from build123d import *

# Parameters (mm, degrees)
F0_R     = 43.4000447198
F1_DEPTH = 110.744
F2_T     = -5.08
F3_R     = 63.6187489092
F4_DEPTH = 5.842
F5_R     = 5.07999
F6_W     = 2.7671808675
F6_H     = 25.928324776
F7_DEPTH = 50.8


# Not quite as in the source:
# - a fillet or chamfer is up to 0.001 mm smaller than in the source, because OpenCascade refuses the exact size


with BuildPart() as f1:
    # F0 (on Top) → F1 (new body)
    with BuildSketch(Plane.XY):
        Circle(F0_R)
    extrude(amount=F1_DEPTH)

    # F2
    f2_openings = [f1.faces().sort_by_distance(p)[0] for p in [
        (0, 0, 110.744),
    ]]
    offset(amount=F2_T, openings=f2_openings)

    # F3 (on Top) → F4 (join)
    with BuildSketch(Plane.XY):
        Circle(F3_R)
    extrude(amount=F4_DEPTH)

    # F5 (radius 5.08 in the source; OpenCascade refuses exactly that, so slightly less here)
    f5_edges = [f1.edges().sort_by_distance(p)[0] for p in [
        (-43.400045, 0, 110.744),
    ]]
    fillet(f5_edges, radius=F5_R)

    # F6 (on Top) → F7 (join)
    with BuildSketch(Plane.XY):
        with BuildLine():
            ThreePointArc((22.0028883346, -9.7789997235), (23.5536000152, -4.9983854371), (24.0781214104, 0))
            ThreePointArc((24.0781214104, 0), (23.5424460635, 5.0506597592), (21.9592547789, 9.8765915281))
            Line((21.9592547789, 9.8765915281), (21.9592547789, -9.7789997235))
            Line((21.9592547789, -9.7789997235), (22.0028883346, -9.7789997235))
        make_face()
        with BuildLine():
            ThreePointArc((21.9592547789, 9.8765915281), (23.5424460635, 5.0506597592), (24.0781214104, 0))
            ThreePointArc((24.0781214104, 0), (23.5536000152, -4.9983854371), (22.0028883346, -9.7789997235))
            Line((22.0028883346, -9.7789997235), (24.7264356464, -9.7789997235))
            Line((24.7264356464, -9.7789997235), (24.7264356464, 16.1493250525))
            Line((24.7264356464, 16.1493250525), (21.9592547789, 16.1493250525))
            Line((21.9592547789, 16.1493250525), (21.9592547789, 9.8765915281))
        make_face()
        with BuildLine():
            Line((21.9592547789, -9.7789997235), (21.9592547789, 9.8765915281))
            ThreePointArc((21.9592547789, 9.8765915281), (2.7373131328, 23.9220201377), (-19.1605677938, 14.5817890698))
            Line((-19.1605677938, 14.5817890698), (-19.1165860754, 14.5817890698))
            Line((-19.1165860754, 14.5817890698), (-19.1165860754, 4.2168572654))
            Line((-19.1165860754, 4.2168572654), (-6.283051686, 4.2168572654))
            Line((-6.283051686, 4.2168572654), (-6.283051686, 14.5817890698))
            Line((-6.283051686, 14.5817890698), (-3.4518897579, 14.5817890698))
            Line((-3.4518897579, 14.5817890698), (-3.4518897579, -9.7789997235))
            Line((-3.4518897579, -9.7789997235), (-6.283051686, -9.7789997235))
            Line((-6.283051686, -9.7789997235), (-6.283051686, 1.6842736198))
            Line((-6.283051686, 1.6842736198), (-19.1165860754, 1.6842736198))
            Line((-19.1165860754, 1.6842736198), (-19.1165860754, -9.7789997235))
            Line((-19.1165860754, -9.7789997235), (-21.9477480035, -9.7789997235))
            Line((-21.9477480035, -9.7789997235), (-21.9477480035, 9.9021355389))
            ThreePointArc((-21.9477480035, 9.9021355389), (-9.8406062526, -21.9754044158), (22.0028883346, -9.7789997235))
            Line((22.0028883346, -9.7789997235), (21.9592547789, -9.7789997235))
        make_face()
        with BuildLine():
            add(Edge.make_bspline(
                [(13.6843709515, -9.837649029), (12.3780909659, -10.1149002912), (10.5279719658, -10.1149002912)],
                knots=[0, 0, 0, 1, 1, 1], degree=2))
            add(Edge.make_bspline(
                [(10.5279719658, -10.1149002912), (6.4811698879, -10.1149002912), (4.1378635463, -7.6462977061)],
                knots=[0, 0, 0, 1, 1, 1], degree=2))
            add(Edge.make_bspline(
                [(4.1378635463, -7.6462977061), (1.7945572048, -5.177695121), (1.7945572048, -0.8003242304)],
                knots=[0, 0, 0, 1, 1, 1], degree=2))
            add(Edge.make_bspline(
                [(1.7945572048, -0.8003242304), (1.7945572048, 3.6197007006), (3.9699132625, 6.2189312842)],
                knots=[0, 0, 0, 1, 1, 1], degree=2))
            add(Edge.make_bspline(
                [(3.9699132625, 6.2189312842), (6.1452693202, 8.8181618679), (9.81351679, 8.8181618679)],
                knots=[0, 0, 0, 1, 1, 1], degree=2))
            add(Edge.make_bspline(
                [(9.81351679, 8.8181618679), (13.2418352829, 8.8181618679), (15.2412434242, 6.560163607)],
                knots=[0, 0, 0, 1, 1, 1], degree=2))
            add(Edge.make_bspline(
                [(15.2412434242, 6.560163607), (17.2406515655, 4.3021653461), (17.2406515655, 0.601927346)],
                knots=[0, 0, 0, 1, 1, 1], degree=2))
            Line((17.2406515655, 0.601927346), (17.2406515655, -1.1468883082))
            Line((17.2406515655, -1.1468883082), (4.6630414181, -1.1468883082))
            add(Edge.make_bspline(
                [(4.6630414181, -1.1468883082), (4.7483494988, -4.3619365994), (6.2892267063, -6.0281100505)],
                knots=[0, 0, 0, 1, 1, 1], degree=2))
            add(Edge.make_bspline(
                [(6.2892267063, -6.0281100505), (7.8301039139, -7.6942835015), (10.6292753117, -7.6942835015)],
                knots=[0, 0, 0, 1, 1, 1], degree=2))
            add(Edge.make_bspline(
                [(10.6292753117, -7.6942835015), (13.5777358507, -7.6942835015), (16.4568835741, -6.4626480865)],
                knots=[0, 0, 0, 1, 1, 1], degree=2))
            Line((16.4568835741, -6.4626480865), (16.4568835741, -8.9312506716))
            add(Edge.make_bspline(
                [(16.4568835741, -8.9312506716), (14.9906509372, -9.5603977667), (13.6843709515, -9.837649029)],
                knots=[0, 0, 0, 1, 1, 1], degree=2))
        make_face(mode=Mode.SUBTRACT)
        with BuildLine():
            Line((-19.1165860754, 14.5817890698), (-19.1605677938, 14.5817890698))
            ThreePointArc((-19.1605677938, 14.5817890698), (-20.6869088124, 12.3210281406), (-21.9477480035, 9.9021355389))
            Line((-21.9477480035, 9.9021355389), (-21.9477480035, -9.7789997235))
            Line((-21.9477480035, -9.7789997235), (-19.1165860754, -9.7789997235))
            Line((-19.1165860754, -9.7789997235), (-19.1165860754, 1.6842736198))
            Line((-19.1165860754, 1.6842736198), (-6.283051686, 1.6842736198))
            Line((-6.283051686, 1.6842736198), (-6.283051686, -9.7789997235))
            Line((-6.283051686, -9.7789997235), (-3.4518897579, -9.7789997235))
            Line((-3.4518897579, -9.7789997235), (-3.4518897579, 14.5817890698))
            Line((-3.4518897579, 14.5817890698), (-6.283051686, 14.5817890698))
            Line((-6.283051686, 14.5817890698), (-6.283051686, 4.2168572654))
            Line((-6.283051686, 4.2168572654), (-19.1165860754, 4.2168572654))
            Line((-19.1165860754, 4.2168572654), (-19.1165860754, 14.5817890698))
        make_face()
        with BuildLine():
            ThreePointArc((-21.9477480035, 9.9021355389), (-20.6869088124, 12.3210281406), (-19.1605677938, 14.5817890698))
            Line((-19.1605677938, 14.5817890698), (-21.9477480035, 14.5817890698))
            Line((-21.9477480035, 14.5817890698), (-21.9477480035, 9.9021355389))
        make_face()
        with Locations((31.9749566279, 3.1851626645)):
            Rectangle(F6_W, F6_H)
        with BuildLine():
            add(Edge.make_bspline(
                [(54.9841455177, -0.629708069), (54.9841455177, -5.0977187954), (52.7368107669, -7.6063095433)],
                knots=[0, 0, 0, 1, 1, 1], degree=2))
            add(Edge.make_bspline(
                [(52.7261472568, 6.2669170796), (54.9841455177, 3.7156722913), (54.9841455177, -0.629708069)],
                knots=[0, 0, 0, 1, 1, 1], degree=2))
            add(Edge.make_bspline(
                [(46.6399488748, 8.8181618679), (50.4681489959, 8.8181618679), (52.7261472568, 6.2669170796)],
                knots=[0, 0, 0, 1, 1, 1], degree=2))
            add(Edge.make_bspline(
                [(40.4391177593, 6.3255663851), (42.6731231225, 8.8181618679), (46.6399488748, 8.8181618679)],
                knots=[0, 0, 0, 1, 1, 1], degree=2))
            add(Edge.make_bspline(
                [(38.2051123961, -0.629708069), (38.2051123961, 3.8329709023), (40.4391177593, 6.3255663851)],
                knots=[0, 0, 0, 1, 1, 1], degree=2))
            add(Edge.make_bspline(
                [(39.2394728745, -5.66288483), (38.2051123961, -3.5141875475), (38.2051123961, -0.629708069)],
                knots=[0, 0, 0, 1, 1, 1], degree=2))
            add(Edge.make_bspline(
                [(42.1719381484, -8.9632412019), (40.2738333529, -7.8115821125), (39.2394728745, -5.66288483)],
                knots=[0, 0, 0, 1, 1, 1], degree=2))
            add(Edge.make_bspline(
                [(46.5226502638, -10.1149002912), (44.0700429438, -10.1149002912), (42.1719381484, -8.9632412019)],
                knots=[0, 0, 0, 1, 1, 1], degree=2))
            add(Edge.make_bspline(
                [(52.7368107669, -7.6063095433), (50.4894760161, -10.1149002912), (46.5226502638, -10.1149002912)],
                knots=[0, 0, 0, 1, 1, 1], degree=2))
        make_face()
        with BuildLine():
            add(Edge.make_bspline(
                [(41.0735966094, -0.629708069), (41.0735966094, -4.1326711325), (42.4731823083, -5.9641289899)],
                knots=[0, 0, 0, 1, 1, 1], degree=2))
            add(Edge.make_bspline(
                [(42.4571870432, 4.6833858317), (41.0735966094, 2.8999137697), (41.0735966094, -0.629708069)],
                knots=[0, 0, 0, 1, 1, 1], degree=2))
            add(Edge.make_bspline(
                [(46.5546407941, 6.4668578937), (43.840777477, 6.4668578937), (42.4571870432, 4.6833858317)],
                knots=[0, 0, 0, 1, 1, 1], degree=2))
            add(Edge.make_bspline(
                [(50.7134097279, 4.659392934), (49.3058263964, 6.4668578937), (46.5546407941, 6.4668578937)],
                knots=[0, 0, 0, 1, 1, 1], degree=2))
            add(Edge.make_bspline(
                [(52.1209930594, -0.629708069), (52.1209930594, 2.8519279743), (50.7134097279, 4.659392934)],
                knots=[0, 0, 0, 1, 1, 1], degree=2))
            add(Edge.make_bspline(
                [(50.7134097279, -5.9721266225), (52.1209930594, -4.1486663977), (52.1209930594, -0.629708069)],
                knots=[0, 0, 0, 1, 1, 1], degree=2))
            add(Edge.make_bspline(
                [(46.5866313243, -7.7955868474), (49.3058263964, -7.7955868474), (50.7134097279, -5.9721266225)],
                knots=[0, 0, 0, 1, 1, 1], degree=2))
            add(Edge.make_bspline(
                [(42.4731823083, -5.9641289899), (43.8727680072, -7.7955868474), (46.5866313243, -7.7955868474)],
                knots=[0, 0, 0, 1, 1, 1], degree=2))
        make_face(mode=Mode.SUBTRACT)
    extrude(amount=F7_DEPTH)


solid = f1.part
Geometry: final body of the model. Coordinates: model frame, mm. A direction names the side the tool comes from. Give positions to 0.01 mm unless a question says otherwise; leave off trailing zeros. Order: outer loops, then holes, each group sorted by start corner. A loop starts at its lowest first (then second) coordinate and runs counter-clockwise, first axis right, second up. Notation, with made-up numbers: (24, 7.5) -> (77, 7.5) arc R19 cw to (77, 15.5) -> close; hole circle Ø2 at (14.5, -9.75). An arc over 180 degrees is marked (long way). Put each result on its own line as item: value.
Q1. Reachability of faces 1 (the face through (-8.31, -37.41, 57.56)), 2 (the face through (-1, 1, 0)) from +Z, -Z, +X, -X, +Y, -Y: full face, straight path, thin tool, end or side. Return the list, or none.
Here are the results:
face 1: +Z
face 2: -Z, +X, -X, +Y, -Y
Q2. Material intervals for L1, parallel to Y at x = 0, z = 37.5; L2, parallel to X at y = 0, z = 35; L3, parallel to Y at x = 0, z = 73.5, sorted ascending.
Here are the results:
L1: y = -43.4 to -38.32, -24.08 to 24.08, 38.32 to 43.4
L2: x = -43.4 to -38.32, -24.08 to 1.81, 17.24 to 24.73, 30.59 to 33.36, 38.22 to 43.4, 52.11 to 54.97
L3: y = -43.4 to -38.32, 38.32 to 43.4
Q3. Section B-B, the plane z = 95. Return loops of the section in (x, y).
Here are the results:
outline: circle Ø86.8 at (0, 0); hole circle Ø76.64 at (0, 0)
Q4. Draft query along X for faces 3 (the face through (53, -1, 50.8)), 4 (the face through (30.591, 3, 28)), 5 (the face through (3.08, 23.88, 28.01)). Return one class per face: released by +X, released by -X, zero draft, split by the parting line, or undercut.
Here are the results:
face 3: zero draft
face 4: undercut
face 5: undercut
Q5. Pin query (flat end, axial travel): pin 1 (3 mm diameter, centred on x = 31.5, z = 38, fed in from +Y); pin 2 (3 mm diameter, centred on y = 15.5, z = 71, fed in from +X); pin 3 (8 mm diameter, centred on y = -19.5, z = 46, fed in from +X). Return the tip coordinate at first contact, or that it passes through.
Here are the results:
pin 1: stops at y = 31.36
pin 2: stops at x = 41.08
pin 3: stops at x = 40.54
